Check sheet for the modelled part. Datum: model origin and axes. Units: mm. Round coordinates to 2 decimals unless told otherwise and drop trailing zeros. Order: outer loops, then holes, each group sorted by start corner. A loop starts at its lowest first (then second) coordinate and runs counter-clockwise, first axis right, second up. Notation, with made-up numbers: (-23, 47) -> (36, 47) arc R21 cw to (36, 86) -> close; hole circle Ø5 at (26.25, -27.75). An arc over 180 degrees is marked (long way). Answer in a Markdown table with one row per item.
Autodesk Inventor part; units mm, degrees
ref_plane "YZ Plane" through (0, 0, 0) normal (1, 0, 0) x (0, 1, 0)
ref_plane "XZ Plane" through (0, 0, 0) normal (0, 1, 0) x (-1, 0, 0)
ref_plane "XY Plane" through (0, 0, 0) normal (0, 0, 1) x (1, 0, 0)
sketch "Boceto1" plane through (0, 0, 0) normal (0, 0, 1) x (1, 0, 0)
  line L0 (-20, 50) -> (5, 50)
  line L1 (20, 35) -> (20, -45)
  line L2 (15, -50) -> (-20, -50)
  line L3 (-20, -50) -> (-20, 50)
  line L4 (0, 26.3033) -> (0, -44.8052)
  line L5 (-41.9778, 0) -> (28.2031, 0)
  arc A0 (20, 35) -> (5, 50) centre (5, 35) ccw
  arc A1 (15, -50) -> (20, -45) centre (15, -45) ccw
  point P0 (0, 0)
  point P1 (0, 50)
  point P2 (-20, 0)
  dimension "d3" = 30
  dimension "d4" = 10
  dimension "d5" = 100
  dimension "d6" = 40
extrude "Extrusión1" add sketch "Boceto1" along normal blind 2
sketch "Boceto2" plane through (0, 0, 2) normal (0, 0, 1) x (1, 0, 0)
  line L0 (-20, -50) -> (15, -50)
  line L1 (20, -45) -> (20, 35)
  line L2 (5, 50) -> (-20, 50)
  line L3 (-20, 50) -> (-20, -50)
  circle A0 centre (-10, 47.5) radius 1
  circle A1 centre (17.5, 35) radius 1
  circle A2 centre (17.5, 15) radius 1
  circle A3 centre (17.5, -5) radius 1
  circle A4 centre (17.5, -25) radius 1
  circle A5 centre (17.5, -45) radius 1
  circle A6 centre (-15, -47.5) radius 1
  point P0 (0, 0)
  dimension "d9" = 2.5
  dimension "d10" = 5
  dimension "d11" = 5
  dimension "d12" = 2.5
  dimension "d13" = 2.5
  dimension "d14" = 2.5
  dimension "d15" = 2.5
  dimension "d16" = 2.5
  dimension "d17" = 10
  dimension "d18" = 20
  dimension "d19" = 20
  dimension "d20" = 20
  dimension "d21" = 2.5
  dimension "d22" = 20
  dimension "d23" = 2
  dimension "d24" = 2
  dimension "d25" = 2
  dimension "d26" = 2
  dimension "d27" = 2
  dimension "d28" = 2
  dimension "d29" = 2
extrude "Extrusión2" [suppressed]
sketch "Boceto3" plane through (0, 0, 0) normal (0, 0, -1) x (-1, 0, 0)
  line L0 (20, -50) -> (20, 50)
  line L1 (20, 50) -> (-5, 50)
  point P0 (0, 0)
  point P1 (-3, 37)
  dimension "d32" = 23
  dimension "d33" = 13
hole "Agujero1" at (3, 37, 0) direction (0, 0, 1) diameter 10 end through all
sketch "Boceto4" plane through (0, 0, 0) normal (0, 0, 1) x (1, 0, 0)
  line L0 (-8.1395, 25) -> (-9.1395, 25)
  line L1 (-9.1395, 25) -> (-9.1395, -25)
  line L2 (-9.1395, -25) -> (-8.1395, -25)
  line L3 (-8.1395, -25) -> (-8.1395, 25)
  line L4 (-48.3206, 0) -> (41.5333, 0)
  line L5 (-4.1395, 25) -> (-5.1395, 25)
  line L6 (-5.1395, 25) -> (-5.1395, -25)
  line L7 (-5.1395, -25) -> (-4.1395, -25)
  line L8 (-4.1395, -25) -> (-4.1395, 25)
  line L9 (-0.1395, 25) -> (-1.1395, 25)
  line L10 (-1.1395, 25) -> (-1.1395, -25)
  line L11 (-1.1395, -25) -> (-0.1395, -25)
  line L12 (-0.1395, -25) -> (-0.1395, 25)
  line L13 (3.8605, 25) -> (2.8605, 25)
  line L14 (2.8605, 25) -> (2.8605, -25)
  line L15 (2.8605, -25) -> (3.8605, -25)
  line L16 (3.8605, -25) -> (3.8605, 25)
  line L17 (7.8605, 25) -> (6.8605, 25)
  line L18 (6.8605, 25) -> (6.8605, -25)
  line L19 (6.8605, -25) -> (7.8605, -25)
  line L20 (7.8605, -25) -> (7.8605, 25)
  point P0 (0, 0)
  point P1 (-9.1395, 0)
  dimension "d41" = 1
  dimension "d42" = 50
  dimension "d43" = 1
  dimension "d44" = 50
  dimension "d45" = 1
  dimension "d46" = 50
  dimension "d47" = 1
  dimension "d48" = 50
  dimension "d49" = 1
  dimension "d50" = 50
  dimension "d51" = 3
  dimension "d52" = 3
  dimension "d53" = 3
  dimension "d54" = 3
extrude "Extrusión3" cut sketch "Boceto4" along normal blind 10
sketch "Boceto5" plane through (0, 0, 0) normal (0, 0, 1) x (1, 0, 0)
  line L0 (5, 50) -> (-20, 50)
  line L1 (20, -45) -> (20, 35)
  line L2 (-20, -50) -> (-20, 50)
  line L3 (2, 63.3665) -> (2, 50)
  line L4 (2, 5) -> (2, -15)
  line L5 (-10, 55.864) -> (-10, 50)
  line L6 (-10, 5) -> (-10, -15)
  line L7 (-56.3903, 5) -> (-20, 5)
  line L8 (-10, 5) -> (2, 5)
  line L9 (20, 5) -> (36.1498, 5)
  line L10 (20, -15) -> (39.7486, -15)
  line L11 (-56.3903, -15) -> (-20, -15)
  line L12 (-10, -15) -> (2, -15)
  point P0 (0, 0)
  dimension "d61" = 10
  dimension "d62" = 20
  dimension "d63" = 45
  dimension "d64" = 12
extrude "Extrusión4" cut sketch "Boceto5" along normal blind 10
sketch "Boceto6" plane through (0, 0, 0) normal (0, 0, 1) x (1, 0, 0)
  line L0 (-10, -15) -> (2, -15)
  line L1 (2, -15) -> (2, 5)
  line L2 (2, 5) -> (-10, 5)
  line L3 (-10, 5) -> (-10, -15)
  line L4 (-12, -17) -> (4, -17)
  line L5 (4, -17) -> (4, 7)
  line L6 (4, 7) -> (-12, 7)
  line L7 (-12, 7) -> (-12, -17)
  point P0 (0, 0)
  point P1 (2, -15)
  point P2 (-10, 5)
  dimension "d67" = 2
extrude "Extrusión5" add sketch "Boceto6" along normal up to surface (2 mm away)
properties part number "base_lateral_cover_rigth_v2" material "Plástico ABS"
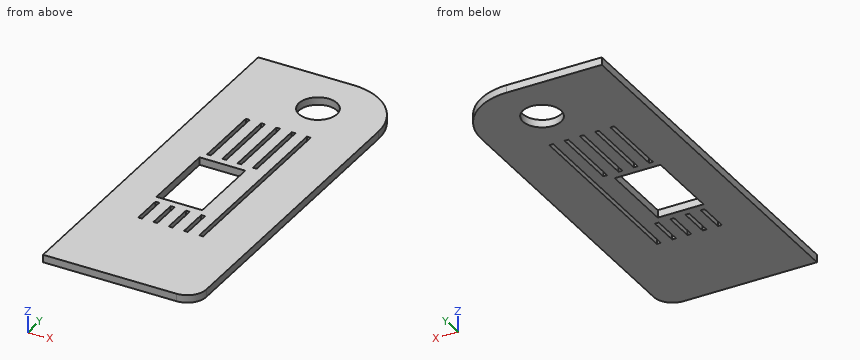
Item 1: Cross-section at B-B (x = 1). Record the boundary of the cut face in (y, z).
Result sheet:
| item | result |
|---|---|
| outline | (-50, 0) -> (-15, 0) -> (-15, 2) -> (-50, 2) -> close; (5, 0) -> (32.42, 0) -> (32.42, 2) -> (5, 2) -> close; (41.58, 0) -> (50, 0) -> (50, 2) -> (41.58, 2) -> close |
Item 2: Cross-section at C-C (y = 37). Record the boundary of the cut face in (x, z), and give its area (3 significant figures).
Result sheet:
| item | result |
|---|---|
| outline | (-20, 0) -> (-2, 0) -> (-2, 2) -> (-20, 2) -> close; (8, 0) -> (19.87, 0) -> (19.87, 2) -> (8, 2) -> close |
| area | 59.7 mm^2 |
Item 3: Cross-section at A-A (y = -24). Record the boundary of the cut face in (x, z), and give its area (3 significant figures).
Result sheet:
| item | result |
|---|---|
| outline | (-20, 0) -> (-9.14, 0) -> (-9.14, 2) -> (-20, 2) -> close; (-8.14, 0) -> (-5.14, 0) -> (-5.14, 2) -> (-8.14, 2) -> close; (-4.14, 0) -> (-1.14, 0) -> (-1.14, 2) -> (-4.14, 2) -> close; (-0.14, 0) -> (2.86, 0) -> (2.86, 2) -> (-0.14, 2) -> close; (3.86, 0) -> (6.86, 0) -> (6.86, 2) -> (3.86, 2) -> close; (7.86, 0) -> (20, 0) -> (20, 2) -> (7.86, 2) -> close |
| area | 70.0 mm^2 |
Item 4: Scan lines: line 1 (Y direction, x = 3, z = 1); line 2 (X direction, y = 7.5, z = 1.6); line 3 (X direction, y = -5.5, z = 0.75). Record each from-to range of solid material in increasing order. Write a range as [from, to].
Result sheet:
| item | result |
|---|---|
| line 1 | y = [-50, -25], [-17, 7], [25, 32], [42, 50] |
| line 2 | x = [-20, -9.14], [-8.14, -5.14], [-4.14, -1.14], [-0.14, 2.86], [3.86, 6.86], [7.86, 20] |
| line 3 | x = [-20, -10], [2, 6.86], [7.86, 20] |
